Build history of the part. All positions in model axes, mm. A direction names the side the tool comes from. Coordinates: 2 decimals unless noted, no trailing zeros. Write each loop counter-clockwise with the first axis right and the second up, starting at its lowest first coordinate (ties: lowest second). Pieces come first, ordered by that corner, then holes.
```python
from build123d import *

# Parameters (mm, degrees)
SKETCH1_W            = 12
SKETCH1_H            = 60
BOSS_EXTRUDE1_DEPTH  = 1
SKETCH4_W            = 12
SKETCH4_H            = 60
BOSS_EXTRUDE5_DEPTH  = 4
SKETCH3_W            = 0.442585723
SKETCH3_H            = 46.400729484
SKETCH3_W_2          = 0.4
CUT_EXTRUDE1_DEPTH   = 3
BOSS_EXTRUDE6_DEPTH  = 7
BOSS_EXTRUDE11_DEPTH = 8
BOSS_EXTRUDE12_DEPTH = 2
BOSS_EXTRUDE13_DEPTH = 0.75
BOSS_EXTRUDE15_DEPTH = 2


with BuildPart() as part:
    # Sketch1 → Boss-Extrude1 (new body)
    with BuildSketch(Plane(origin=(0, 0, 0), x_dir=(1, 0, 0), z_dir=(0, 1, 0))):
        with Locations((-1.342029662, -10.461538462)):
            Rectangle(SKETCH1_W, SKETCH1_H)
    extrude(amount=BOSS_EXTRUDE1_DEPTH)

    # Sketch4 → Boss-Extrude5 (add)
    with BuildSketch(Plane(origin=(0, 0, 0), x_dir=(1, 0, 0), z_dir=(0, 1, 0))):
        with Locations((-1.342029662, -10.461538462)):
            Rectangle(SKETCH4_W, SKETCH4_H)
        Polygon((-2.096130055, -33.457130572), (-6.384615385, -37.75443168), (-6.384611455, -29.168649172), align=None, mode=Mode.SUBTRACT)
        Polygon((2.908277834, -38.461538462), (-5.677508603, -38.461538462), (-1.384615385, -34.168645243), align=None, mode=Mode.SUBTRACT)
        Polygon((-1.38975443, -32.749302861), (-5.677336591, -28.461186458), (-1.384615385, -24.168121227), (2.898997747, -28.451734358), align=None, mode=Mode.SUBTRACT)
        Polygon((-2.091498793, -23.461237818), (-6.384610808, -27.754427103), (-6.384606877, -19.168129734), align=None, mode=Mode.SUBTRACT)
        Polygon((-1.384401984, -22.754128282), (-5.676963509, -18.461572954), (-1.384618257, -14.16814285), (2.90844487, -18.461204162), align=None, mode=Mode.SUBTRACT)
        Polygon((-2.094846949, -13.457914458), (-6.38460623, -17.742175237), (-6.38460623, -9.168156991), align=None, mode=Mode.SUBTRACT)
        Polygon((3.615384615, -29.168645243), (3.615384615, -37.75443168), (-0.749170508, -33.533200366), align=None, mode=Mode.SUBTRACT)
        Polygon((3.615384615, -19.168465252), (3.615384615, -27.753907665), (-0.677336591, -23.461186458), align=None, mode=Mode.SUBTRACT)
        Polygon((3.615384615, -17.754251693), (-0.676897524, -13.461506969), (3.615384615, -9.169224829), align=None, mode=Mode.SUBTRACT)
        Polygon((-6.384597723, 0.832144172), (-2.091409836, -3.461043715), (-6.384601653, -7.753916614), align=None, mode=Mode.SUBTRACT)
        Polygon((2.908517821, -8.460971372), (-1.387204346, -12.751178894), (-5.677010576, -8.461229413), (-1.384615385, -4.167838166), align=None, mode=Mode.SUBTRACT)
        Polygon((-1.385221722, -2.75490806), (-5.679497842, 1.537745361), (-1.38541394, 5.831829263), (2.908210299, 1.538205024), align=None, mode=Mode.SUBTRACT)
        Polygon((-2.089578329, 6.535993652), (-6.3837953, 2.241776681), (-6.384597078, 2.240974904), (-6.384597078, 2.242578156), (-6.384593146, 10.83100847), align=None, mode=Mode.SUBTRACT)
        Polygon((-5.677832652, 11.538461538), (2.912889557, 11.538461538), (-1.382471548, 7.243100433), align=None, mode=Mode.SUBTRACT)
        Polygon((3.615384615, -7.755011267), (-0.677821818, -3.462040655), (3.615384615, 0.831165778), align=None, mode=Mode.SUBTRACT)
        Polygon((3.615384615, 2.245379341), (-0.678307159, 6.538936044), (3.615384615, 10.832627818), align=None, mode=Mode.SUBTRACT)
    extrude(amount=-BOSS_EXTRUDE5_DEPTH)

    # Sketch3 → Cut-Extrude1 (cut)
    with BuildSketch(Plane.XZ.offset(4)):
        with Locations((3.436677476, 13.26117372)):
            Rectangle(SKETCH3_W, SKETCH3_H)
        with Locations((-6.184615385, 13.26117372)):
            Rectangle(SKETCH3_W_2, SKETCH3_H)
    extrude(amount=-CUT_EXTRUDE1_DEPTH, mode=Mode.SUBTRACT)

    # Sketch5 → Boss-Extrude6 (add)
    with BuildSketch(Plane(origin=(0, 0, -19.538461538), x_dir=(-1, 0, 0), z_dir=(0, 0, -1))):
        Polygon((-12.288789064, 5.355892869), (14.972848388, 5.355892869), (3.537352374, -9.415920613), (1.425918842, -12.033387248), (-0.689767913, -9.409188123), align=None)
        with BuildLine():
            Line((9.692725832, 1.966121199), (9.999443939, 1.857726092))
            Line((9.999443939, 1.857726092), (10.306162047, 1.966121199))
            ThreePointArc((10.306162047, 1.966121199), (9.999443939, 3.917921599), (9.692725832, 1.966121199))
        make_face(mode=Mode.SUBTRACT)
        with BuildLine():
            Line((-7.622102723, 1.966121199), (-7.315384615, 1.857726092))
            Line((-7.315384615, 1.857726092), (-7.008666508, 1.966121199))
            ThreePointArc((-7.008666508, 1.966121199), (-7.315384615, 3.917921599), (-7.622102723, 1.966121199))
        make_face(mode=Mode.SUBTRACT)
        with BuildLine():
            Line((0.921478569, 1.79402802), (1.342029662, 1.636661499))
            Line((1.342029662, 1.636661499), (1.762580755, 1.79402802))
            ThreePointArc((1.762580755, 1.79402802), (1.342029662, 4.117921599), (0.921478569, 1.79402802))
        make_face(mode=Mode.SUBTRACT)
    extrude(amount=-BOSS_EXTRUDE6_DEPTH)

    # Sketch5<3> → Boss-Extrude11 (add)
    with BuildSketch(Plane(origin=(0, 0, -19.538461538), x_dir=(-1, 0, 0), z_dir=(0, 0, -1))):
        with BuildLine():
            Line((3.537352374, -9.415920613), (1.425918842, -12.033387248))
            Line((1.425918842, -12.033387248), (-0.689767913, -9.409188123))
            ThreePointArc((-0.689767913, -9.409188123), (1.429900561, -5.57732435), (3.537352374, -9.415920613))
        make_face()
    extrude(amount=BOSS_EXTRUDE11_DEPTH)

    # Sketch11 → Boss-Extrude12 (add)
    with BuildSketch(Plane.ZY.offset(7.342029662)):
        Polygon((-12.538461538, 5.355892869), (-4.993833778, 1), (-12.538461538, 1), align=None)
    extrude(amount=-BOSS_EXTRUDE12_DEPTH)

    # Sketch12 → Boss-Extrude13 (add, symmetric)
    with BuildSketch(Plane.ZY.offset(1.342029662)):
        Polygon((-13.859142787, 0.316720052), (-13.859142787, -4.418628297), (-13.859142787, -9.68323793), (-6.410996577, -3.888931374), (-6.410996577, 0.316720052), align=None)
    extrude(amount=BOSS_EXTRUDE13_DEPTH, both=True)

    # Sketch14 → Boss-Extrude15 (add)
    with BuildSketch(Plane(origin=(4.657970338, 0, 0), x_dir=(0, 0, -1), z_dir=(1, 0, 0))):
        Polygon((4.993833778, 1), (12.538461538, 5.355892869), (12.538461538, 1), align=None)
    extrude(amount=-BOSS_EXTRUDE15_DEPTH)


solid = part.part
```
1. 3-axis set-ups, long thin cutter, end or side, ignore diameter. For faces 1 (the face through (-2.3, 4.2, -12.538)), 2 (the face through (-3.5, -1.97, 10.64)), 3 (the face through (-10.039, 3.917, -16.087)): which of +Z, -Z, +X, -X, +Y, -Y reach the whole face in a straight line?
Computed values:
face 1: +Z, +Y
face 2: -Y
face 3: +Z, -Z
2. Saw through at A-A on z = -13.5. List the corners of the cut face in (x, y).
Computed values:
outline: (-14.97, 5.36) - (-3.54, -9.42) - (-1.43, -12.03) - (0.69, -9.41) - (12.29, 5.36) - close; hole (-10.31, 1.97) - (-10, 1.86) - (-9.69, 1.97) arc R1 ccw (long way) to start; hole (-1.76, 1.79) - (-1.34, 1.64) - (-0.92, 1.79) arc R1.2 ccw (long way) to start; hole (7.01, 1.97) - (7.32, 1.86) - (7.62, 1.97) arc R1 ccw (long way) to start
3. Flat gauge pins, fed straight in: pin 1 (3 mm diameter, centred on x = -9.5, y = 0, fed in from +Z); pin 2 (8 mm diameter, centred on x = -8.5, z = -3, fed in from -Y); pin 3 (4.5 mm diameter, centred on y = 0, z = 12.5, fed in from -X); pin 4 (1.5 mm diameter, centred on x = -5, y = -9.5, fed in from +Z). Where does each tip first touch, or does it go through?
Computed values:
pin 1: stops at z = -12.54
pin 2: stops at y = -4
pin 3: stops at x = -7.34
pin 4: passes through
4. Probe line 1 along X through (y, z) = (-2.25, 0); line 2 along X through (y, z) = (-1.5, 8); line 3 along X through (y, z) = (-0.75, -11.5). List the from-to ranges inside material, lowest first.
Computed values:
line 1: x = -7.34 to -6.38, -5.55 to -4.14, 1.37 to 2.78, 3.66 to 4.66
line 2: x = -7.34 to -6.38, -5.98 to -5.22, 2.45 to 3.22, 3.66 to 4.66
line 3: x = -7.34 to -5.64, -2.09 to -0.59, 2.87 to 4.66
5. Saw through at C-C on y = -6.5. List the corners of the cut face in (x, z).
Computed values:
outline: (-5.79, -19.54) - (-3.37, -19.54) - (-3.37, -27.54) - (0.51, -27.54) - (0.51, -19.54) - (2.98, -19.54) - (2.98, -12.54) - (-0.59, -12.54) - (-0.59, -9.77) - (-2.09, -9.77) - (-2.09, -12.54) - (-5.79, -12.54) - close
6. Mould opens along X. For faces 4 (the face through (-1, -1, 40.462)), 5 (the face through (1.48, -1.97, -8.7)), 6 (the face through (-1.36, -5.58, -23.48)) say: +X half, -X half, draft (parallel to the pull), parting line (faces both ways), or undercut.
Computed values:
face 4: draft
face 5: undercut
face 6: parting line
7. Saw through at D-D on x = 10.25. List the corners of the cut face in (y, z).
Computed values:
outline: (2.76, -19.54) - (5.36, -19.54) - (5.36, -12.54) - (2.76, -12.54) - close
